```python
from build123d import *

# Parameters (mm, degrees)
SKETCH1_W           = 99.695
SKETCH1_H           = 60.198
BOSS_EXTRUDE1_DEPTH = 24.384
SKETCH2_R           = 26.2255
BOSS_EXTRUDE2_DEPTH = 4.318
SKETCH3_R           = 3.429
BOSS_EXTRUDE3_DEPTH = 1.27
SKETCH4_R           = 3.556
SKETCH4_R_2         = 5.842
SKETCH4_R_3         = 7.3025
BOSS_EXTRUDE4_DEPTH = 0.635
SKETCH7_R           = 2.54
CUT_EXTRUDE1_DEPTH  = 0.508
SKETCH8_R           = 3.175
CUT_EXTRUDE2_DEPTH  = 6.604
SKETCH9_W           = 10.16
SKETCH9_H           = 51.816
BOSS_EXTRUDE5_DEPTH = 6.35
SKETCH10_W          = 16.726375359
SKETCH10_H          = 49.657
BOSS_EXTRUDE6_DEPTH = 6.35
SKETCH11_R          = 30.734
BOSS_EXTRUDE7_DEPTH = 101.6


with BuildPart() as part:
    # Sketch1 → Boss-Extrude1 (new body)
    with BuildSketch(Plane.XY):
        with Locations((49.8475, 30.099)):
            Rectangle(SKETCH1_W, SKETCH1_H)
    extrude(amount=BOSS_EXTRUDE1_DEPTH)

    # Sketch2 → Boss-Extrude2 (add)
    with BuildSketch(Plane.XY.offset(24.384)):
        with Locations(Location((59.758770255, 29.6545, 0), (0, 0, 180))):
            Circle(SKETCH2_R)
    extrude(amount=BOSS_EXTRUDE2_DEPTH)

    # Sketch3 → Boss-Extrude3 (add)
    with BuildSketch(Plane.XY.offset(24.384)):
        with Locations(Location((86.106, 10.16, 0), (0, 0, 180))):
            Circle(SKETCH3_R)
    extrude(amount=BOSS_EXTRUDE3_DEPTH)

    # Sketch4 → Boss-Extrude4 (add)
    with BuildSketch(Plane(origin=(0, 60.198, 0), x_dir=(1, 0, 0), z_dir=(0, 1, 0))):
        with Locations(Location((10.414, -16.256, 0), (0, 0, 90))):
            Circle(SKETCH4_R)
        with Locations(Location((23.749, -16.256, 0), (0, 0, 90))):
            Circle(SKETCH4_R_2)
        with Locations(Location((42.545, -9.652, 0), (0, 0, 90))):
            Circle(SKETCH4_R_3)
    extrude(amount=BOSS_EXTRUDE4_DEPTH)

    # Sketch7 → Cut-Extrude1 (cut)
    with BuildSketch(Plane(origin=(0, 60.198, 0), x_dir=(1, 0, 0), z_dir=(0, 1, 0))):
        with Locations(Location((34.163, -19.304, 0), (0, 0, 270))):
            Circle(SKETCH7_R)
    extrude(amount=-CUT_EXTRUDE1_DEPTH, mode=Mode.SUBTRACT)

    # Sketch8 → Cut-Extrude2 (cut)
    with BuildSketch(Plane.XZ):
        with Locations(Location((60.325, 14.224, 0), (0, 0, 270))):
            Circle(SKETCH8_R)
    extrude(amount=-CUT_EXTRUDE2_DEPTH, mode=Mode.SUBTRACT)

    # Sketch9 → Boss-Extrude5 (add)
    with BuildSketch(Plane.ZY):
        with Locations((13.97, 27.94)):
            Rectangle(SKETCH9_W, SKETCH9_H)
    extrude(amount=BOSS_EXTRUDE5_DEPTH)

    # Sketch10 → Boss-Extrude6 (add)
    with BuildSketch(Plane(origin=(99.695, 0, 0), x_dir=(0, 0, -1), z_dir=(1, 0, 0))):
        with Locations((-11.15718768, 29.0195)):
            Rectangle(SKETCH10_W, SKETCH10_H)
    extrude(amount=BOSS_EXTRUDE6_DEPTH)

    # Sketch11 → Boss-Extrude7 (add)
    with BuildSketch(Plane.XY.offset(28.702)):
        with Locations((59.758770255, 29.6545)):
            Circle(SKETCH11_R)
    extrude(amount=BOSS_EXTRUDE7_DEPTH)


solid = part.part
```
Can you work these out from the model? Positions are in its coordinate system, mm. A direction names the side the tool comes from. Coordinates: 2 decimals unless noted, no trailing zeros. Loops run counter-clockwise (first coordinate to the right, second up) from the corner with the lowest first, then second, coordinate; pieces in that order, holes last. Notation, with made-up numbers: (73, -29.75) -> (117, -29.75) arc R27 cw to (117, -6.75) -> close; hole circle Ø5 at (19, 62.5). An arc over 180 degrees is marked (long way). Put each result on its own line as item: value. Start each with the question number.
Q1. I want a section at D-D (z = 117). Write out the boundary of the cut face in (x, y), plus the area to 3 significant figures.
Q2. I want a section at B-B (x = 3). Write out the boundary of the cut face in (y, z), plus the area to 3 significant figures.
Q3. Thinking about a two-plate mould opening in X: for faces 5 (the face through (60, 6.604, 14)), 6 (the face through (35.37, 10.95, 78.79)), 7 (the face through (-3, 28, 8.89)), which applies, pulls with the +X half, pulls with the -X half, needs draft (parallel to the pull), parting line crosses it, or undercut?
Q4. I'm going to push flat-ended pins straight in: P1, Ø7, axis at x = -4.5, z = 14, coming from the +Y side; P2, Ø5, axis at y = 33.5, z = 115, coming from the +X side; P3, Ø3, axis at x = 59.5, z = 13, coming from the -Y side. Where does each tip first touch, or does it pass through?
Q5. If I drill on line 1 (Z direction, x = 97.5, y = 47); line 2 (Z direction, x = 50, y = 55); line 3 (Y direction, x = 91, z = 12), over which ranges is the centre line in solid material (lowest first)? Write a range as [from, to].
Q6. I want a section at A-A (y = 39). Write out the boundary of the cut face in (x, z) (3 decimals).
Q7. I want a section at C-C (y = 27). Write out the boundary of the cut face in (x, z) (3 decimals).
Q8. For faces 1 (the face through (103, 4.191, 11)), 2 (the face through (63.002, 3.256, 12.517)), 3 (the face through (103, 29, 19.52)), 4 (the face through (35.305, 60.511, 10.603)), which set-ups out of +Z, -Z, +X, -X, +Y, -Y let a thin tool reach every point of the face, with its end or its side?
Taken from the geometry:
1. outline: circle Ø61.47 at (59.76, 29.65)
1. area: 2,970 mm2
2. outline: (0, 0) -> (60.2, 0) -> (60.2, 24.38) -> (0, 24.38) -> close
2. area: 1,470 mm2
3. face 5: undercut
3. face 6: parting line crosses it
3. face 7: needs draft
4. P1: stops at y = 53.85
4. P2: stops at x = 90.46
4. P3: stops at y = 6.6
5. line 1: z = [0, 24.38]
5. line 2: z = [0, 24.38], [28.7, 130.3]
5. line 3: y = [0, 60.2]
6. outline: (-6.35, 8.89) -> (0, 8.89) -> (0, 0) -> (99.695, 0) -> (99.695, 2.794) -> (106.045, 2.794) -> (106.045, 19.52) -> (99.695, 19.52) -> (99.695, 24.384) -> (84.263, 24.384) -> (84.263, 28.702) -> (89.037, 28.702) -> (89.037, 130.302) -> (30.48, 130.302) -> (30.48, 28.702) -> (35.255, 28.702) -> (35.255, 24.384) -> (0, 24.384) -> (0, 19.05) -> (-6.35, 19.05) -> close
7. outline: (-6.35, 8.89) -> (0, 8.89) -> (0, 0) -> (99.695, 0) -> (99.695, 2.794) -> (106.045, 2.794) -> (106.045, 19.52) -> (99.695, 19.52) -> (99.695, 24.384) -> (85.85, 24.384) -> (85.85, 28.702) -> (90.378, 28.702) -> (90.378, 130.302) -> (29.14, 130.302) -> (29.14, 28.702) -> (33.668, 28.702) -> (33.668, 24.384) -> (0, 24.384) -> (0, 19.05) -> (-6.35, 19.05) -> close
8. face 1: +Z, -Z, +X, -Y
8. face 2: -Y
8. face 3: +Z, +X, +Y, -Y
8. face 4: +Y
